```python
from build123d import *

# Parameters (mm, degrees)
BOSS_EXTRUDE1_DEPTH  = 9.15
SKETCH4_W            = 52.35
SKETCH4_H            = 5.35
CUT_EXTRUDE2_DEPTH   = 3
SKETCH6_R            = 2.725
BOSS_EXTRUDE2_DEPTH  = 13.65
SKETCH8_R            = 1.5
BOSS_EXTRUDE3_DEPTH  = 8.75
SKETCH9_R            = 1.6
BOSS_EXTRUDE4_DEPTH  = 4.6
SKETCH10_R           = 2.6
SKETCH10_R_2         = 0.925
BOSS_EXTRUDE5_DEPTH  = 7.55
SKETCH11_W           = 12.15
SKETCH11_H           = 6
BOSS_EXTRUDE6_DEPTH  = 1.9
BOSS_EXTRUDE7_DEPTH  = 4.75
SKETCH13_R           = 2.05
BOSS_EXTRUDE8_DEPTH  = 9.425
FILLET1_R            = 0.5
BOSS_EXTRUDE9_DEPTH  = 9.15
SKETCH20_R           = 2.725
BOSS_EXTRUDE10_DEPTH = 1.55
SKETCH21_R           = 1.5
CUT_EXTRUDE3_DEPTH   = 3


with BuildPart() as part:
    # Sketch1 → Boss-Extrude1 (new body)
    with BuildSketch(Plane.XY):
        Polygon((0, 0), (54.25, 0), (54.25, 4.6), (44.52, 4.6), (44.52, 8.9), (42.25, 8.9), (42.25, 4.6), (16.1, 4.6), (0, 3.25), align=None)
    extrude(amount=-BOSS_EXTRUDE1_DEPTH)

    # Sketch4 → Cut-Extrude2 (cut)
    with BuildSketch(Plane.XZ):
        with Locations((28.075, -4.575)):
            Rectangle(SKETCH4_W, SKETCH4_H)
    extrude(amount=-CUT_EXTRUDE2_DEPTH, mode=Mode.SUBTRACT)

    # Sketch6 → Boss-Extrude2 (add)
    with BuildSketch(Plane(origin=(0, 0, -10.65), x_dir=(-1, 0, 0), z_dir=(0, 0, -1))):
        with Locations((-54.25, 2.3)):
            Circle(SKETCH6_R)
    extrude(amount=-BOSS_EXTRUDE2_DEPTH)

    # Sketch8 → Boss-Extrude3 (add)
    with BuildSketch(Plane.XY.offset(-17.9)):
        with Locations((54.25, 2.3)):
            Circle(SKETCH8_R)
    extrude(amount=BOSS_EXTRUDE3_DEPTH)

    # Sketch9 → Boss-Extrude4 (add)
    with BuildSketch(Plane.XY.offset(3)):
        with Locations((54.25, 2.3)):
            Circle(SKETCH9_R)
    extrude(amount=BOSS_EXTRUDE4_DEPTH)

    # Sketch10 → Boss-Extrude5 (add)
    with BuildSketch(Plane.XZ.offset(-3)):
        with Locations((20.95, -5.325)):
            Circle(SKETCH10_R)
        with Locations((20.95, -5.325)):
            Circle(SKETCH10_R_2, mode=Mode.SUBTRACT)
    extrude(amount=BOSS_EXTRUDE5_DEPTH)

    # Sketch11 → Boss-Extrude6 (add)
    with BuildSketch(Plane.XY):
        with Locations((24.825, -3)):
            Rectangle(SKETCH11_W, SKETCH11_H)
    extrude(amount=-BOSS_EXTRUDE6_DEPTH)

    # Sketch12 → Boss-Extrude7 (add)
    with BuildSketch(Plane.XY):
        Polygon((24.7, -6), (24.7, -2.5), (23.5, -2.5), (22.15, -3.9), (22.15, -6), align=None)
    extrude(amount=BOSS_EXTRUDE7_DEPTH)

    # Sketch13 → Boss-Extrude8 (add)
    with BuildSketch(Plane(origin=(54.3, 0, 0), x_dir=(0, 0, -1), z_dir=(1, 0, 0))):
        with Locations((4.575, 2.3)):
            Circle(SKETCH13_R)
    extrude(amount=BOSS_EXTRUDE8_DEPTH)

    # Fillet1
    fillet1_edges = [part.edges().sort_by_distance(p)[0] for p in [
        (0, 1.625, 0),
        (0, 1.625, -9.15),
    ]]
    fillet(fillet1_edges, radius=FILLET1_R)

    # Sketch19 → Boss-Extrude9 (add)
    with BuildSketch(Plane.XY):
        Polygon((0.5, 0), (-1.2, 0), (-1.2, 3.149378882), (0.5, 3.291925466), align=None)
    extrude(amount=-BOSS_EXTRUDE9_DEPTH)

    # Sketch20 → Boss-Extrude10 (add)
    with BuildSketch(Plane.XY.offset(3)):
        with Locations((54.25, 2.3)):
            Circle(SKETCH20_R)
    extrude(amount=BOSS_EXTRUDE10_DEPTH)

    # Sketch21 → Cut-Extrude3 (cut)
    with BuildSketch(Plane(origin=(0, 0, -17.9), x_dir=(-1, 0, 0), z_dir=(0, 0, -1))):
        with Locations((-54.25, 2.3)):
            Circle(SKETCH21_R)
    extrude(amount=-CUT_EXTRUDE3_DEPTH, mode=Mode.SUBTRACT)


solid = part.part
```
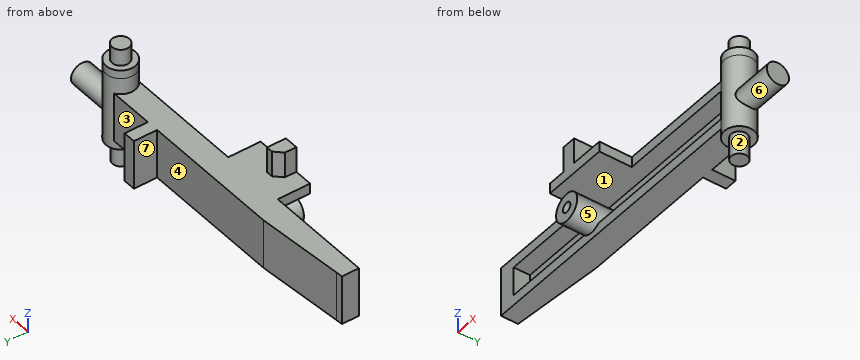
Input: part model. Units: mm. Frame: model coordinates. Face numbers are marked on the shaded views. A direction names the side the tool comes from. Give positions to 0.01 mm unless a question says otherwise; leave off trailing zeros. Write each loop counter-clockwise with the first axis right and the second up, starting at its lowest first coordinate (ties: lowest second). Pieces come first, ordered by that corner, then holes. Notation, with made-up numbers: (-30.75, 55.25) - (-14.75, 55.25) arc R21 cw to (-14.75, 63.25) - close; hole circle Ø7 at (16.5, -16). An arc over 180 degrees is marked (long way). Write item = value, one per line. Start each with the question number.
1. Ray query, L1, parallel to Z at x = 20.95, y = -2.25 (3 decimals); L2, parallel to Z at x = 20.95, y = 0.25 (3 decimals); L3, parallel to Z at x = 41, y = 2.25. Return the intervals inside material, ascending.
2. Section query A-A, the plane x = 54.25. Output: boundary loops of the cut face in (y, z) (3 decimals).
3. Mould query, pull axis Z, two halves, no side actions, for the marked faces 5, 6 and 7. Classes: released by +Z, released by -Z, zero draft, split by the parting line, or undercut.
4. First-contact query: pin 1 Ø2.5 at (x, y) = (14.5, -1.5) entering from -Z; pin 2 Ø1.3 at (x, y) = (23, -4.5) entering from +Z; pin 3 Ø5 at (x, z) = (32.5, -6.5) entering from -Y; pin 4 Ø0.6 at (x, z) = (21, -5.5) entering from -Y. Flat tips, straight axial feed; report the tip coordinate or a pass-through.
5. Section query C-C, the plane y = 5.75. Output: boundary loops of the cut face in (x, z), then the cut area to 3 significant figures.
6. Section query B-B, the plane y = -1.5. Output: boundary loops of the cut face in (x, z) (3 decimals).
7. Section query D-D, the plane x = 29. Output: boundary loops of the cut face in (y, z), then the cut area to 3 significant figures.
8. Access query for the marked faces 1, 2, 3 and 4. Directions: +Z, -Z, +X, -X, +Y, -Y. A direction counts if a zero-diameter tool reaches every point of the face in a straight line with its end or side. Return the directions, or none.
Check sheet entries:
q1.L1 = -7.925 to -6.25, -4.4 to -2.725, -1.9 to 0
q1.L2 = -9.15 to -6.25, -4.4 to -2.725, -1.9 to 0
q1.L3 = -9.15 to -7.25, -1.9 to 0
q2.outline = (-0.425, -10.65) - (0.8, -10.65) - (0.8, -14.9) - (3.8, -14.9) - (3.8, -10.65) - (5.025, -10.65) - (5.025, 4.55) - (3.9, 4.55) - (3.9, 7.6) - (0.7, 7.6) - (0.7, 4.55) - (-0.425, 4.55) - close
q3.face_5 = undercut
q3.face_6 = split by the parting line
q3.face_7 = zero draft
q4.pin_1 = through
q4.pin_2 = 4.75
q4.pin_3 = 0
q4.pin_4 = 3
q5.outline = (42.25, -9.15) - (44.52, -9.15) - (44.52, 0) - (42.25, 0) - close
q5.area = 20.8 mm2
q6.outline = circle Ø5.2 at (20.95, -5.325); (18.75, -1.9) - (30.9, -1.9) - (30.9, 0) - (18.75, 0) - close; hole circle Ø1.85 at (20.95, -5.325)
q7.outline = (-6, -1.9) - (3, -1.9) - (3, -7.25) - (0, -7.25) - (0, -9.15) - (4.6, -9.15) - (4.6, 0) - (-6, 0) - close
q7.area = 37.4 mm2
q8.face_1 = -Y
q8.face_2 = -Z
q8.face_3 = +Z, -Z, +Y
q8.face_4 = +Z, -Z, -X, +Y
